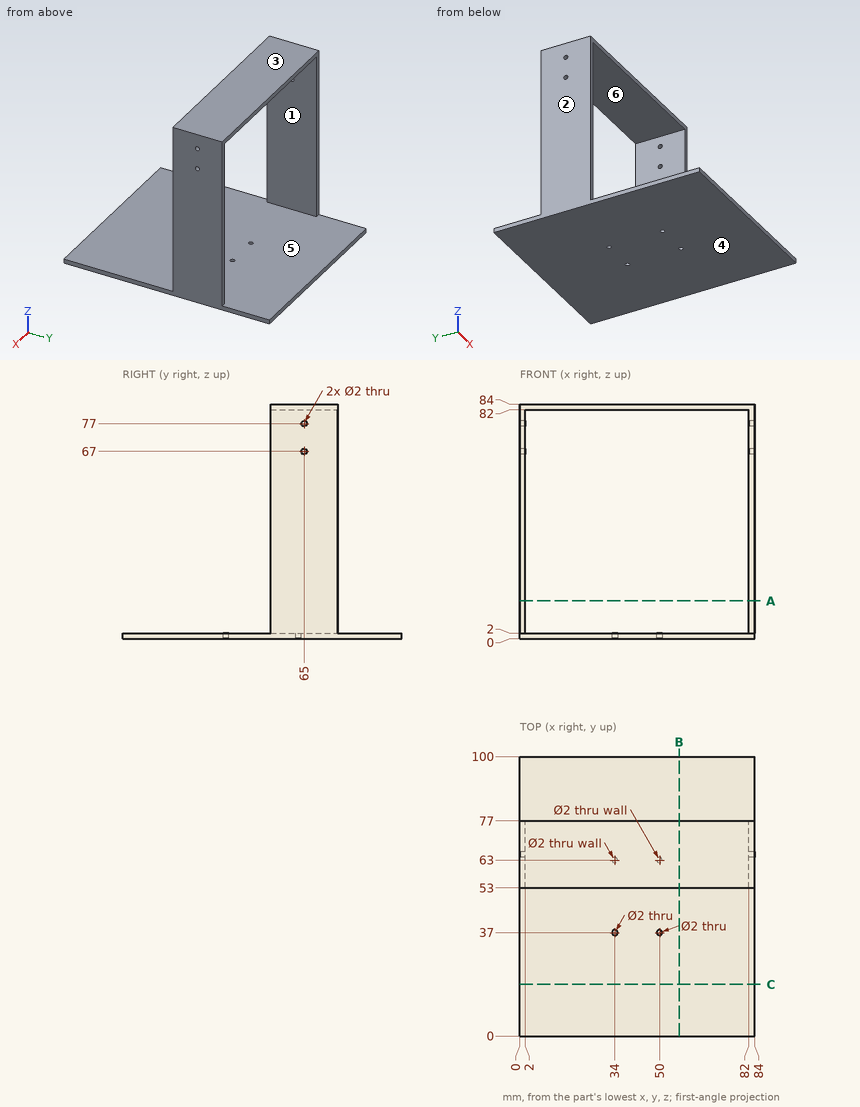
The drawing under review shows one solid part. Ordinate dimensions are in mm from its lowest x, y, z. A direction names the side the tool comes from. Round coordinates to 2 decimals unless told otherwise and drop trailing zeros. Loops run counter-clockwise (first coordinate to the right, second up) from the corner with the lowest first, then second, coordinate; pieces in that order, holes last. Notation, with made-up numbers: (4.25, 87.25) - (21.25, 87.25) arc R23 cw to (21.25, 122.25) - close; hole circle Ø8 at (17, 83). An arc over 180 degrees is marked (long way). One line per question, with ' | ' between items.
Q1. The part is to be moulded in two halves that separate along Z. For the marked faces 3, 4, 5 and 6, say which applies: released by +Z, released by -Z, zero draft, split by the parting line, or undercut.
Taken from the geometry:
face 3: released by +Z | face 4: released by -Z | face 5: undercut | face 6: undercut
Q2. Take a section at A-A (z = 13.5). Give the boundary of the cut face in (x, y).
Taken from the geometry:
outline: (0, 53) - (2, 53) - (2, 77) - (0, 77) - close; (82, 53) - (84, 53) - (84, 77) - (82, 77) - close
Q3. Take a section at B-B (x = 57). Give the boundary of the cut face in (y, z).
Taken from the geometry:
outline: (0, 0) - (100, 0) - (100, 2) - (0, 2) - close; (53, 82) - (77, 82) - (77, 84) - (53, 84) - close
Q4. Tool access review of the marked faces 1 and 2: name each direction out of +Z, -Z, +X, -X, +Y, -Y from which nothing blocks a thin tool from reaching the whole face with its end or side.
Taken from the geometry:
face 1: +Y, -Y | face 2: +Z, -Z, -X, +Y, -Y
Q5. For line 1 along X through (y, z) = (63, 1.25); line 2 along Y through (x, z) = (50, 1); line 3 along Z through (x, y) = (0.5, 65), list the stretches that pass through material, from the lowest coordinate up. Write a range as [from, to].
Taken from the geometry:
line 1: x = [0, 33], [35, 49], [51, 84] | line 2: y = [0, 36], [38, 62], [64, 100] | line 3: z = [0, 66], [68, 76], [78, 84]
Q6. Take a section at C-C (y = 18.5). Give the boundary of the cut face in (x, z), and give its area (3 significant figures).
Taken from the geometry:
outline: (0, 0) - (84, 0) - (84, 2) - (0, 2) - close | area: 168 mm²
Q7. For pin 1 (1.8 mm diameter, centred on x = 50, y = 37, fed in from -Z); pin 2 (12 mm diameter, centred on x = 35.5, y = 42, fed in from -Z), all flat-tipped, find the tip position at first contact; note any pin that passes through.
Taken from the geometry:
pin 1: passes through | pin 2: stops at z = 0
